Source: CAD feature listing. Evaluate the final solid. Frame: model axes, mm. Face numbers are marked on the shaded views. A direction names the side the tool comes from. Coordinates: 2 decimals unless noted, no trailing zeros. Order: outer loops, then holes, each group sorted by start corner. A loop starts at its lowest first (then second) coordinate and runs counter-clockwise, first axis right, second up.
```python
from build123d import *

# Parameters (mm, degrees)
SKETCH3_W           = 30
SKETCH3_H           = 6
BOSS_EXTRUDE2_DEPTH = 5
SKETCH4_W           = 4
SKETCH4_H           = 6
BOSS_EXTRUDE3_DEPTH = 17
SKETCH7_R           = 1.5
CUT_EXTRUDE2_DEPTH  = 50
SKETCH9_W           = 5
SKETCH9_H           = 6
BOSS_EXTRUDE5_DEPTH = 8
SKETCH10_R          = 1.35
CUT_EXTRUDE3_DEPTH  = 8
SKETCH11_W          = 2
SKETCH11_H          = 2
CUT_EXTRUDE4_DEPTH  = 8
FILLET2_R           = 3


with BuildPart() as part:
    # Sketch3 → Boss-Extrude2 (new body)
    with BuildSketch(Plane(origin=(0, 0, 0), x_dir=(1, 0, 0), z_dir=(0, 1, 0))):
        Rectangle(SKETCH3_W, SKETCH3_H)
    extrude(amount=BOSS_EXTRUDE2_DEPTH)

    # Sketch4 → Boss-Extrude3 (add)
    with BuildSketch(Plane(origin=(0, 5, 0), x_dir=(1, 0, 0), z_dir=(0, 1, 0))):
        with Locations((-13, 0)):
            Rectangle(SKETCH4_W, SKETCH4_H)
        with Locations((13, 0)):
            Rectangle(SKETCH4_W, SKETCH4_H)
    extrude(amount=BOSS_EXTRUDE3_DEPTH)

    # Sketch7 → Cut-Extrude2 (cut, symmetric)
    with BuildSketch(Plane.ZY.offset(-11)):
        with Locations((0, 15)):
            Circle(SKETCH7_R)
    extrude(amount=CUT_EXTRUDE2_DEPTH, both=True, mode=Mode.SUBTRACT)

    # Sketch9 → Boss-Extrude5 (add)
    with BuildSketch(Plane.XZ):
        with Locations((-8.5, 0)):
            Rectangle(SKETCH9_W, SKETCH9_H)
        with Locations((8.5, 0)):
            Rectangle(SKETCH9_W, SKETCH9_H)
    extrude(amount=BOSS_EXTRUDE5_DEPTH)

    # Sketch10 → Cut-Extrude3 (cut)
    with BuildSketch(Plane(origin=(11, 0, 0), x_dir=(0, 0, -1), z_dir=(1, 0, 0))):
        with Locations((0, -5)):
            Circle(SKETCH10_R)
    extrude(amount=-CUT_EXTRUDE3_DEPTH, mode=Mode.SUBTRACT)

    # Sketch11 → Cut-Extrude4 (cut)
    with BuildSketch(Plane.ZY.offset(11)):
        with Locations((0, -5)):
            Rectangle(SKETCH11_W, SKETCH11_H)
    extrude(amount=-CUT_EXTRUDE4_DEPTH, mode=Mode.SUBTRACT)

    # Fillet2
    fillet2_edges = [part.edges().sort_by_distance(p)[0] for p in [
        (-8.5, -8, -3),
        (8.5, -8, -3),
        (8.5, -8, 3),
        (-8.5, -8, 3),
    ]]
    fillet(fillet2_edges, radius=FILLET2_R - 0.0001)  # a hair under: the kernel refuses the full size


solid = part.part
```
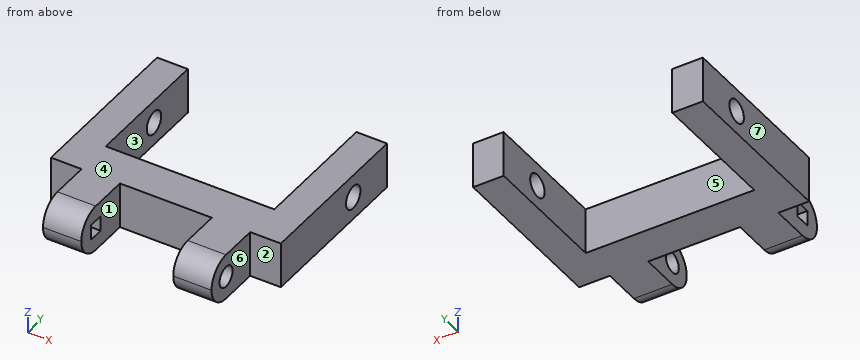
1. Section query D-D on z = -0.5. Count the separate pieces of the cut face and the enclosed holes in it, plus the area to 3 significant figures.
Findings:
separate pieces: 5
enclosed holes: 0
area: 320 mm2
2. Access query for the marked faces 1, 2 and 3. Directions: +Z, -Z, +X, -X, +Y, -Y. A direction counts if a zero-diameter tool reaches every point of the face in a straight line with its end or side. Return the directions, or none.
Findings:
face 1: +Z, -Z, -Y
face 2: +Z, -Z, +X, -Y
face 3: +Z, -Z, +Y
3. Draft query along X for the marked faces 4, 5, 6 and 7. Return one class per face: released by +X, released by -X, zero draft, split by the parting line, or undercut.
Findings:
face 4: zero draft
face 5: undercut
face 6: released by +X
face 7: released by -X
4. Pin query (flat end, axial travel): P1, Ø2.5, axis at y = 15, z = 0, coming from the +X side; P2, Ø1, axis at x = -8.5, z = -0.5, coming from the +Y side; P3, Ø1.8, axis at x = -1, z = 1.5, coming from the -Y side; P4, Ø3, axis at y = -5, z = -0.5, coming from the -X side. Return the tip coordinate at first contact, or that it passes through.
Findings:
P1: passes through
P2: stops at y = 5
P3: stops at y = 0
P4: stops at x = -11
5. Section query B-B on y = 15. Return loops of the section in (x, z), plus the area to 3 significant figures.
Findings:
outline: (-15, -3) - (-11, -3) - (-11, -1.5) - (-15, -1.5) - close; (-15, 1.5) - (-11, 1.5) - (-11, 3) - (-15, 3) - close; (11, -3) - (15, -3) - (15, -1.5) - (11, -1.5) - close; (11, 1.5) - (15, 1.5) - (15, 3) - (11, 3) - close
area: 24.0 mm2
6. Ray query, line 1 (Y direction, x = -14, z = 0); line 2 (Y direction, x = 7.45, z = 0); line 3 (X direction, y = 8.5, z = 2.5). Return the intervals inside material, ascending.
Findings:
line 1: y = 0 to 13.5, 16.5 to 22
line 2: y = -8 to -6.35, -3.65 to 5
line 3: x = -15 to -11, 11 to 15
7. Section query A-A on y = -0.5. Return loops of the section in (x, z).
Findings:
outline: (-11, -3) - (-6, -3) - (-6, 3) - (-11, 3) - close; (6, -3) - (11, -3) - (11, 3) - (6, 3) - close
